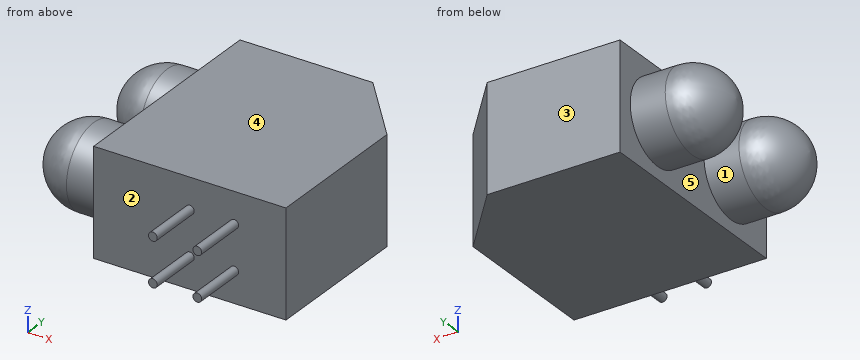
Autodesk Inventor part; units mm, degrees
ref_plane "Work Plane1" through (0, 0, 3.05) normal (0, 0, 1) x (1, 0, 0)
ref_plane "Work Plane2" through (0, 6.195, 0) normal (0, 1, 0) x (1, 0, 0)
ref_plane "YZ Plane" through (0, 0, 0) normal (1, 0, 0) x (0, 1, 0)
sketch "Sketch1" plane through (0, 0, 0) normal (0, 0, 1) x (1, 0, 0)
  line L0 (0, 0) -> (11, 0)
  line L1 (11, 0) -> (11, 8.7)
  line L2 (0, 0) -> (0, 12.6)
  line L3 (0, 12.6) -> (7.6, 12.6)
  line L4 (7.6, 12.6) -> (11, 8.7)
  dimension "d0" = 11
  dimension "d1" = 8.7
  dimension "d2" = 12.6
  dimension "d3" = 7.6
extrude "Extrusion1" add sketch "Sketch1" along normal blind 6.1
ref_plane "Work Plane1" through (0, 0, 3.05) normal (0, 0, 1) x (1, 0, 0)
sketch "Sketch2" plane through (0, 0, 3.05) normal (0, 0, 1) x (1, 0, 0)
  line L0 (0, 12.6) -> (0, 0)
  line L1 (0, 9.37) -> (-4.5, 9.37)
  line L2 (7.6, 12.6) -> (0, 12.6)
  line L3 (0, 11.72) -> (-2, 11.72)
  arc A0 (-2, 11.72) -> (-4.5, 9.37) centre (-2, 9.2152) ccw
  line L4 (0, 9.37) -> (0, 11.72)
  line L5 (0, 12.6) -> (0, 0)
  dimension "d6" = 3.23
  dimension "d7" = 4.5
  dimension "d8" = 2.35
  dimension "d10" = 2
revolve "Revolution1" add sketch "Sketch2" angle 360 about axis through (0, 9.37, 3.05) along (-1, 0, 0)
ref_plane "Work Plane2" through (0, 6.195, 0) normal (0, 1, 0) x (1, 0, 0)
mirror "Mirror1" about plane through (0, 6.195, 0) normal (0, 1, 0) of "Revolution1"
sketch "Sketch3" plane through (0, 0, 0) normal (0, -1, 0) x (1, 0, 0)
  circle A0 centre (5.5, 1.78) radius 0.25
  line L0 (0, 0) -> (0, 6.1)
  line L1 (0, 0) -> (11, 0) construction
  line L2 (0, 0) -> (11, 0)
  circle A1 centre (8.04, 1.78) radius 0.25
  line L3 (2.54, 0) -> (13.54, 0)
  circle A2 centre (5.5, 4.32) radius 0.25
  line L4 (0, 2.54) -> (11, 2.54)
  circle A3 centre (8.04, 4.32) radius 0.25
  line L5 (2.54, 2.54) -> (13.54, 2.54)
  point P0 (0, 3.05)
  point P1 (0, 3.05)
  dimension "d13" = 5.5
  dimension "d15" = 1.27
  dimension "d16" = 0.5
  dimension "d19" = 2.54
  dimension "d22" = 2.54
extrude "Extrusion2" add sketch "Sketch3" along normal blind 3.18
properties part number "SSF-LXHM250GGD"
Geometry: final body of the model. Coordinates: model frame, mm. Face numbers are marked on the shaded views. A direction names the side the tool comes from. Coordinates: 2 decimals unless noted, no trailing zeros. Write each loop counter-clockwise with the first axis right and the second up, starting at its lowest first coordinate (ties: lowest second). Pieces come first, ordered by that corner, then holes. Notation, with made-up numbers: (72.5, 28) - (92.5, 28) arc R15 cw to (92.5, 42) - close; hole circle Ø7 at (28.25, 25). An arc over 180 degrees is marked (long way). Return JSON: item names as keys, results as strings.
Item 1: Pin query (flat end, axial travel): pin 1 Ø2 at (x, z) = (-2.5, 4.5) entering from -Y; pin 2 Ø1.8 at (y, z) = (5.5, 2) entering from -X. Return the tip coordinate at first contact, or that it passes through.
Completed:
{"pin 1": "stops at y = 0.73", "pin 2": "stops at x = -3.57"}
Item 2: Section query B-B (x = 8.04). Output: boundary loops of the cut face in (y, z).
Completed:
{"outline": "(-3.18, 1.53) - (0, 1.53) - (0, 0) - (12.1, 0) - (12.1, 6.1) - (0, 6.1) - (0, 4.57) - (-3.18, 4.57) - (-3.18, 4.07) - (0, 4.07) - (0, 2.03) - (-3.18, 2.03) - close"}
Item 3: Reachability of the marked faces 4 and 5 from +Z, -Z, +X, -X, +Y, -Y: full face, straight path, thin tool, end or side. Return the list, or none.
Completed:
{"face 4": "+Z, +X, -X, +Y, -Y", "face 5": "-X"}
Item 4: Section query C-C (x = 2.5). Output: boundary loops of the cut face in (y, z).
Completed:
{"outline": "(0, 0) - (12.6, 0) - (12.6, 6.1) - (0, 6.1) - close"}
Item 5: Line query: L1, parallel to X at y = 6, z = 1; L2, parallel to Y at x = 1.25, z = 5.25; L3, parallel to Y at x = -2.75, z = 1.25. Output: solid intervals per line, ascending.
Completed:
{"L1": "x = 0 to 11", "L2": "y = 0 to 12.6", "L3": "y = 1.7 to 4.34, 8.05 to 10.69"}
Item 6: Pull-direction query (Y, two-part tool) for the marked faces 1, 2 and 3; classes: +Y half, -Y half, draft (parallel to the pull), parting line (faces both ways), or undercut.
Completed:
{"face 1": "undercut", "face 2": "-Y half", "face 3": "+Y half"}
Item 7: Section query A-A (y = -1). Output: boundary loops of the cut face in (x, z).
Completed:
{"outline": "circle Ø0.5 at (5.5, 1.78); circle Ø0.5 at (5.5, 4.32); circle Ø0.5 at (8.04, 1.78); circle Ø0.5 at (8.04, 4.32)"}
